Geometry check sheet. Reference: the model listing, model coordinates, mm. A direction names the side the tool comes from. Coordinates: 2 decimals unless noted, no trailing zeros. Loops run counter-clockwise (first coordinate to the right, second up) from the corner with the lowest first, then second, coordinate; pieces in that order, holes last. Notation, with made-up numbers: M 83,-25.5 L 90,-25.5 A23 cw 90,-17.5 Z; hole C -14.75,55.5 d1. An arc over 180 degrees is marked long. One line per question, with ' | ' between items. Start each with the question number.
Autodesk Inventor part; units mm, degrees
ref_plane "YZ Plane" through (0, 0, 0) normal (1, 0, 0) x (0, 1, 0)
ref_plane "XZ Plane" through (0, 0, 0) normal (0, 1, 0) x (-1, 0, 0)
ref_plane "XY Plane" through (0, 0, 0) normal (0, 0, 1) x (1, 0, 0)
sketch "Esquisse1" plane through (0, 0, 0) normal (1, 0, 0) x (0, 1, 0)
  line L0 (0, 52) -> (3, 52)
  line L1 (3, 32) -> (4, 32)
  line L2 (4, 32) -> (4, 15)
  line L3 (4, 0) -> (3, 0)
  line L4 (3, 0) -> (3, -6)
  line L5 (3, -6) -> (0, -6)
  line L6 (0, 64.5811) -> (0, -64.5811)
  line L7 (4, 15) -> (5, 15)
  line L8 (5, 15) -> (5, 13)
  line L9 (5, 13) -> (4, 13)
  line L10 (4, 13) -> (4, 0)
  line L11 (3, 43.5) -> (2.5, 43.5)
  line L12 (2.5, 43.5) -> (2.5, 37)
  line L13 (2.5, 37) -> (3, 37)
  line L14 (3, 37) -> (3, 43.5) construction
  line L15 (3, 52) -> (3, 43.5)
  line L16 (3, 37) -> (3, 32)
  point P0 (0, 0)
  dimension "d1" = 6
  dimension "d3" = 8
  dimension "d4" = 2
  dimension "d5" = 10
  dimension "d6" = 13
  dimension "d7" = 17
  dimension "d8" = 20
  dimension "d9" = 6
  dimension "d16" = 0.5
  dimension "d17" = 8.5
  dimension "d18" = 5
revolve "Révolution1" add sketch "Esquisse1" angle 360 about axis through (0, 0, 64.5811) along (0, 0, -1)
sketch "Esquisse2" plane through (0, 0, 0) normal (1, 0, 0) x (0, 1, 0)
  line L0 (7, 32) -> (3, 32)
  line L1 (3, 32) -> (3, 0)
  line L2 (3, 0) -> (7, 0)
  line L3 (7, 0) -> (7, 32)
  line L4 (-4, 0) -> (4, 0)
  line L5 (-4, 32) -> (4, 32)
  point P0 (0, 0)
  point P1 (0, 0)
  dimension "d11" = 3
  dimension "d12" = 4
extrude "Extrusion1" cut sketch "Esquisse2" along normal through all both and the other way through all
chamfer "Chanfrein1" distance 0.5 angle 45 2 edges at (0, -3, 52) (0, -3, -6)
properties part number "arbre_roue"
1. Depth check by flat-ended pin: pin 1 Ø2 at (y, z) = (-1, 45.5) entering from -X; pin 2 Ø2 at (x, z) = (0, 20.5) entering from -Y. Enter the tip coordinate at first touch or a pass-through.
2. Thickness scan on line 1 (Z direction, x = 4, y = -2.5); line 2 (Z direction, x = -3, y = -1); line 3 (Z direction, x = -1.25, y = 2.25). Record the ranges inside material, lowest first.
3. Draft check along Z on faces 1 (the flat face through (-1, -3, 32)), 2 (the cylindrical face through (0, -4, 6)), 3 (the flat face through (2, -2, 43.5)), 4 (the flat face through (0, 0, -6)). Enter one of: +Z half, -Z half, draft (parallel to the pull), parting line (faces both ways), or undercut.
4. Sectioned sample at C-C (z = -0.5). Record the cut outline in (x, y).
5. Tool access check on faces 5 (the flat face through (2, -2, 37)), 6 (the cylindrical face through (0, -4, 23)), 7 (the flat face through (-1, -3, 0)), 8 (the flat face through (0, 3, 16)). Record the directions out of +Z, -Z, +X, -X, +Y, -Y that give a thin tool (end or side, any length) a straight path to the whole face; none if there is none.
6. Sectioned sample at D-D (z = 38). Record the cut outline in (x, y), and give its area (3 significant figures).
7. Sectioned sample at B-B (z = 13.5). Record the cut outline in (x, y).
Result:
1) pin 1: stops at x = -3 | pin 2: stops at y = -4
2) line 1: z = 13 to 15 | line 2: z = 0 to 32 | line 3: z = -5.93 to 37, 43.5 to 51.93
3) face 1: +Z half | face 2: draft | face 3: undercut | face 4: -Z half
4) outline: C 0,0 d6
5) face 5: none | face 6: +Z | face 7: -Z | face 8: +Z, -Z, +X, -X, +Y
6) outline: C 0,0 d5 | area: 19.6 mm2
7) outline: M -4,3 A5 ccw long 4,3 Z
